Work out the finished part from the listing and answer in its coordinate system (mm). A direction names the side the tool comes from. Give positions to 0.01 mm unless a question says otherwise; leave off trailing zeros. Order: outer loops, then holes, each group sorted by start corner. A loop starts at its lowest first (then second) coordinate and runs counter-clockwise, first axis right, second up.
```python
from build123d import *

# Parameters (mm, degrees)
BOSS_EXTRUDE1_DEPTH             = 3.25
CBORE_FOR_M3_SBHCS1_D           = 3.4
CBORE_FOR_M3_SBHCS1_CBORE_D     = 5.7
CBORE_FOR_M3_SBHCS1_CBORE_DEPTH = 2.9
SKETCH6_W                       = 2.9
SKETCH6_H                       = 5.7
CUT_EXTRUDE1_DEPTH              = 42.300847449
M3X0_5_TAPPED_HOLE1_D           = 2.5
M3X0_5_TAPPED_HOLE1_DEPTH       = 8
M3X0_5_TAPPED_HOLE1_TIP         = 0.751075774
FILLET1_R                       = 1


with BuildPart() as part:
    # Sketch1 → Boss-Extrude1 (new, symmetric)
    with BuildSketch(Plane.XY):
        with BuildLine():
            Line((-18.4, 18.4), (-18.4, 0))
            Line((-18.4, 0), (18.4, 0))
            Line((18.4, 0), (18.4, 18.4))
            ThreePointArc((18.4, 18.4), (0, 36.8), (-18.4, 18.4))
        make_face()
        with BuildLine():
            Line((6.25, 25.4), (6.25, 11.4))
            ThreePointArc((6.25, 11.4), (0, 5.15), (-6.25, 11.4))
            Line((-6.25, 11.4), (-6.25, 25.4))
            ThreePointArc((-6.25, 25.4), (0, 31.65), (6.25, 25.4))
        make_face(mode=Mode.SUBTRACT)
    extrude(amount=BOSS_EXTRUDE1_DEPTH, both=True)

    # CBORE for M3 SBHCS1 (through all)
    with Locations(Plane.XY.offset(3.25)):
        with Locations((7.75, 4.976606241), (15.5, 18.4), (7.75, 31.823393759), (-7.75, 31.823393759), (-15.5, 18.4), (-7.75, 4.976606241)):
            CounterBoreHole(CBORE_FOR_M3_SBHCS1_D / 2, CBORE_FOR_M3_SBHCS1_CBORE_D / 2, CBORE_FOR_M3_SBHCS1_CBORE_DEPTH)

    # Sketch6 → Cut-Extrude1 (cut, through all)
    with BuildSketch(Plane.XY.offset(0.35)):
        with Locations((-16.95, 18.4)):
            Rectangle(SKETCH6_W, SKETCH6_H)
        with Locations((16.95, 18.4)):
            Rectangle(SKETCH6_W, SKETCH6_H)
        Polygon((-10.218172401, 30.398393759), (-11.674711226, 32.921193007), (-6.725476951, 35.748867784), (-5.281827599, 33.248393759), align=None)
        Polygon((5.281827599, 33.248393759), (6.731827599, 35.75986743), (11.668172401, 32.90986743), (10.218172401, 30.398393759), align=None)
    extrude(amount=CUT_EXTRUDE1_DEPTH, mode=Mode.SUBTRACT)

    # M3x0.5 Tapped Hole1
    with Locations(Plane(origin=(0, 0, 0), x_dir=(-1, 0, 0), z_dir=(0, -1, 0))):
        with Locations((14.8, 0), (0, 0), (-14.8, 0)):
            Hole(M3X0_5_TAPPED_HOLE1_D / 2, depth=M3X0_5_TAPPED_HOLE1_DEPTH)
            with Locations((0, 0, -(M3X0_5_TAPPED_HOLE1_DEPTH + M3X0_5_TAPPED_HOLE1_TIP / 2))):  # 118° drill point
                Cone(0, M3X0_5_TAPPED_HOLE1_D / 2, M3X0_5_TAPPED_HOLE1_TIP, mode=Mode.SUBTRACT)

    # Fillet1
    fillet1_edges = [part.edges().sort_by_distance(p)[0] for p in [
        (-18.177939927, 21.25, 1.8),
        (-18.4, 15.55, 1.8),
        (11.557142364, 32.717557765, 1.8),
        (6.620797563, 35.567557765, 1.8),
        (-6.620797563, 35.567557765, 1.8),
        (-11.557142364, 32.717557765, 1.8),
        (18.4, 15.55, 1.8),
        (18.177939927, 21.25, 1.8),
    ]]
    fillet(fillet1_edges, radius=FILLET1_R)


solid = part.part
```
1. The part is cut by section C-C (x = 4). Write down the section's boundary in (y, z), then the cut area to 3 significant figures.
Findings below:
outline: (0, -3.25) - (6.6, -3.25) - (6.6, 3.25) - (0, 3.25) - close; (30.2, -3.25) - (36.36, -3.25) - (36.36, 3.25) - (30.2, 3.25) - close
area: 82.9 mm2
2. The part is cut by section A-A (x = 0). Write down the section's boundary in (y, z).
Findings below:
outline: (0, -3.25) - (5.15, -3.25) - (5.15, -1.25) - (0, -1.25) - close; (0, 1.25) - (5.15, 1.25) - (5.15, 3.25) - (0, 3.25) - close; (31.65, -3.25) - (36.8, -3.25) - (36.8, 3.25) - (31.65, 3.25) - close
3. The part is cut by section B-B (y = 28). Write down the section's boundary in (x, z).
Findings below:
outline: (-15.7, -3.25) - (-5.68, -3.25) - (-5.68, 3.25) - (-15.7, 3.25) - close; (5.68, -3.25) - (15.7, -3.25) - (15.7, 3.25) - (5.68, 3.25) - close
4. The part is cut by section D-D (z = -2.25). Write down the section's boundary in (x, y).
Findings below:
outline: (-18.4, 0) - (18.4, 0) - (18.4, 18.4) arc R18.4 ccw to (-18.4, 18.4) - close; hole circle Ø3.4 at (-15.5, 18.4); hole circle Ø3.4 at (-7.75, 4.98); hole circle Ø3.4 at (-7.75, 31.82); hole (-6.25, 11.4) arc R6.25 ccw to (6.25, 11.4) - (6.25, 25.4) arc R6.25 ccw to (-6.25, 25.4) - close; hole circle Ø3.4 at (7.75, 4.98); hole circle Ø3.4 at (7.75, 31.82); hole circle Ø3.4 at (15.5, 18.4)
5. Straight lines are drawn through the part: probe 1 along X at (y, z) = (15, -2.5); probe 2 along Y at (x, z) = (7.75, -2.2); probe 3 along X at (y, z) = (6, -0.75). For each, find the intervals that lie inside material, in ascending order.
Findings below:
probe 1: x = -18.4 to -6.25, 6.25 to 18.4
probe 2: y = 0 to 3.28, 6.68 to 30.12, 33.52 to 35.09
probe 3: x = -18.4 to -15.8, -13.8 to -9.11, -6.39 to -3.15, 3.15 to 6.39, 9.11 to 13.8, 15.8 to 18.4
6. The mould has two halves that part along Y. Classify faces 5 (the face through (-0.3, 0, 1.5)), 6 (the face through (8, 3, 0.35)), 7 (the face through (11.68, 32.16, 1.82)): pulls with the +Y half, pulls with the -Y half, needs draft (parallel to the pull), parting line crosses it, or undercut.
Findings below:
face 5: pulls with the -Y half
face 6: undercut
face 7: pulls with the +Y half
7. Given P1, Ø1.5, axis at x = -12.5, z = -2, coming from the +Y side; P2, Ø1.5, axis at x = 16, z = 2, coming from the +Y side; P3, Ø3.5, axis at x = -9, y = 32.5, coming from the +Z side, each flat-ended and moving along its own axis, determine where each tip first touches the part or whether it passes through.
Findings below:
P1: stops at y = 32.56
P2: stops at y = 28.7
P3: stops at z = 0.35
8. Which of the six approach directions +Z, -Z, +X, -X, +Y, -Y give full straight-line access (tool end or side, diameter ignored) to faces 1 (the face through (10.59, 31.04, 1.78)), 2 (the face through (10, 33, 0.35)), 3 (the face through (6.25, 18, 0)), 4 (the face through (-17.76, 21.64, 1.82))?
Findings below:
face 1: +Z, +Y
face 2: +Z
face 3: +Z, -Z
face 4: +Z, -X
